Autodesk Inventor part; units mm, degrees
ref_plane "YZ Plane" through (0, 0, 0) normal (1, 0, 0) x (0, 1, 0)
ref_plane "XZ Plane" through (0, 0, 0) normal (0, 1, 0) x (-1, 0, 0)
ref_plane "XY Plane" through (0, 0, 0) normal (0, 0, 1) x (1, 0, 0)
sketch "Sketch1" plane through (0, 0, 0) normal (0, 1, 0) x (-1, 0, 0)
  circle A0 centre (0, 0) radius 4.5
  line L0 (0, 0) -> (0, -15)
  circle A1 centre (0, -15) radius 0.5
  circle A2 centre (0, -15) radius 1.5
  line L1 (4.3151, -1.2768) -> (1.4994, -15.0417)
  line L2 (-4.3151, -1.2768) -> (-1.4994, -15.0417)
  circle A3 centre (0, -6) radius 0.5
  circle A4 centre (0, -9) radius 0.5
  circle A5 centre (0, -12) radius 0.5
  line L3 (0, 0) -> (-1.4994, 0)
  circle A6 centre (0, 15) radius 0.5
  circle A7 centre (0, 15) radius 1.5
  line L4 (4.3151, 1.2768) -> (1.4994, 15.0417)
  line L5 (-4.3151, 1.2768) -> (-1.4994, 15.0417)
  circle A8 centre (0, 6) radius 0.5
  circle A9 centre (0, 9) radius 0.5
  circle A10 centre (0, 12) radius 0.5
  circle A11 centre (0, 0) radius 2.5
  circle A12 centre (-6, 0) radius 0.5
  circle A13 centre (-9, 0) radius 0.5
  circle A14 centre (-12, 0) radius 0.5
  circle A15 centre (-15, 0) radius 0.5
  circle A16 centre (-15, 0) radius 1.5
  line L6 (-1.2768, -4.3151) -> (-15.0417, -1.4994)
  line L7 (-1.2768, 4.3151) -> (-15.0417, 1.4994)
  circle A17 centre (0, 6) radius 0.5
  circle A18 centre (0, 9) radius 0.5
  circle A19 centre (0, 12) radius 0.5
  circle A20 centre (0, 15) radius 0.5
  circle A21 centre (0, 15) radius 1.5
  line L8 (-4.3151, 1.2768) -> (-1.4994, 15.0417)
  line L9 (4.3151, 1.2768) -> (1.4994, 15.0417)
  circle A22 centre (6, 0) radius 0.5
  circle A23 centre (9, 0) radius 0.5
  circle A24 centre (12, 0) radius 0.5
  circle A25 centre (15, 0) radius 0.5
  circle A26 centre (15, 0) radius 1.5
  line L10 (1.2768, 4.3151) -> (15.0417, 1.4994)
  line L11 (1.2768, -4.3151) -> (15.0417, -1.4994)
  point P0 (3.7991, -3.7991)
  point P1 (3.7991, 3.7991)
  point P2 (-3.7991, 3.7991)
  point P3 (-15.0417, 1.4994)
  point P4 (-3.7991, -3.7991)
  dimension "d0" = 9
  dimension "d3" = 3
  dimension "d1" = 15
  dimension "d2" = 1
  dimension "d4" = 1
  dimension "d5" = 1
  dimension "d6" = 1
  dimension "d8" = 3
  dimension "d9" = 3
  dimension "d10" = 3
  dimension "d13" = 5
  dimension "d18" = 360
extrude "Extrusion1" add sketch "Sketch1" along normal blind 2.5 contours A0 L4 L10 A26 L11 L1 | A0 L10 L4 | L1 L11 A0 | A0 L7 L5 A7 L4 L10 | L11 L1 A2 L0 A5 A4 A3 A0 | A0 L5 L7 | A7 | A26 | L0 A3 A4 A5 A2 L2 L6 A0 | A2 | A0 L2 L6 A16 L7 L5 | L6 L2 A0 | A16
extrude "Extrusion2" add sketch "Sketch1" along normal blind 5.5 contours A0
properties part number "90Horn"
The listing builds one solid part. Answer for the finished solid, in the listing's coordinates (mm). Coordinates: 2 decimals unless noted, no trailing zeros. Write each loop counter-clockwise with the first axis right and the second up, starting at its lowest first coordinate (ties: lowest second). Pieces come first, ordered by that corner, then holes. Notation, with made-up numbers: M -3,-6.5 L 14,-6.5 A27 cw 14,27.5 Z; hole C -29,-38 d10. An arc over 180 degrees is marked long. Put each result on its own line as item: value. Start each with the question number.
1. Consider line 1 (Z direction, x = 0, y = 3.4); line 2 (Z direction, x = -15, y = 0.35). Determine where each line is inside the solid, lowest interval first. Write a range as from..to.
2. A cutting plane is placed at A-A on y = 1.8. Count the separate pieces of the cut face and the enclosed holes in it, then the cut area to 3 significant figures.
3. For a pull along Z with two mould halves and no side action, classify faces 1 (the cylindrical face through (0.065, 1.232, 14.504)), 2 (the flat face through (-2.665, 1.232, -9.342)), 3 (the cylindrical face through (16.5, 1.2, 0)), 4 (the cylindrical face through (0.108, 1.232, 9.488)) as pulls with the +Z half, pulls with the -Z half, needs draft (parallel to the pull), parting line crosses it, or undercut.
4. A cutting plane is placed at C-C on z = 9. Write down the section's boundary in (x, y), then the cut area to 3 significant figures.
5. A cutting plane is placed at D-D on y = 4.8. Write down the section's boundary in (x, z), then the cut area to 3 significant figures.
6. A cutting plane is placed at B-B on x = 9. Write down the section's boundary in (y, z).
7. Flat-ended cylindrical pins translate along their axes: P1, Ø1.5, axis at x = 7, z = -2.5, coming from the +Y side; P2, Ø3, axis at x = 11.5, y = 3.5, coming from the -Z side; P3, Ø2, axis at y = 4, z = 3, coming from the +X side. Find the tip coordinate at first contact, or state that the pin passes through.
Resolved:
1. line 1: z = -4.5..-2.5, 2.5..4.5
1. line 2: z = -1.51..-0.5, 0.5..1.51
2. separate pieces: 1
2. enclosed holes: 17
2. area: 277 mm2
3. face 1: undercut
3. face 2: pulls with the -Z half
3. face 3: parting line crosses it
3. face 4: undercut
4. outline: M -2.74,0 L -0.5,0 L -0.5,2.5 L -2.74,2.5 Z; M 0.5,0 L 2.74,0 L 2.74,2.5 L 0.5,2.5 Z
4. area: 11.2 mm2
5. outline: C 0,0 d9; hole C 0,0 d5
5. area: 44.0 mm2
6. outline: M 0,-2.74 L 2.5,-2.74 L 2.5,-0.5 L 0,-0.5 Z; M 0,0.5 L 2.5,0.5 L 2.5,2.74 L 0,2.74 Z
7. P1: stops at y = 2.5
7. P2: stops at z = -2.45
7. P3: stops at x = 4.03
